Read the model definition and answer for the solid it produces. Units are mm, in the model's axes. Face numbers are marked on the shaded views. Coordinates: 2 decimals unless noted, no trailing zeros. Loops run counter-clockwise (first coordinate to the right, second up) from the corner with the lowest first, then second, coordinate; pieces in that order, holes last. Notation, with made-up numbers: (20.25, -11) - (30.25, -11) arc R21 ccw to (30.25, 18) - close; hole circle Ø1 at (78, 40.5). An arc over 180 degrees is marked (long way). Use one line per item in the form item = value. Start each with the question number.
1) Each of these flat-tipped pins is pushed along its axis until it touches: P1, Ø10, axis at x = -0.5, y = 4.5, coming from the -Z side; P2, Ø1.5, axis at y = -2.5, z = 3.5, coming from the -X side. Where does it stop, or does it pass through?
2) Consider line 1 (Y direction, x = 0, z = 2.7); line 2 (X direction, y = 2, z = 1.3); line 3 (X direction, y = 4.75, z = 2.05). Determine where each line is inside the solid, lowest interval first.
3) The mould has two halves that part along X. Classify the marked faces 1 and 2: released by +X, released by -X, zero draft, split by the parting line, or undercut.
4) A cutting plane is placed at A-A (y = 0). Give the vertices of the cut face in (x, z).
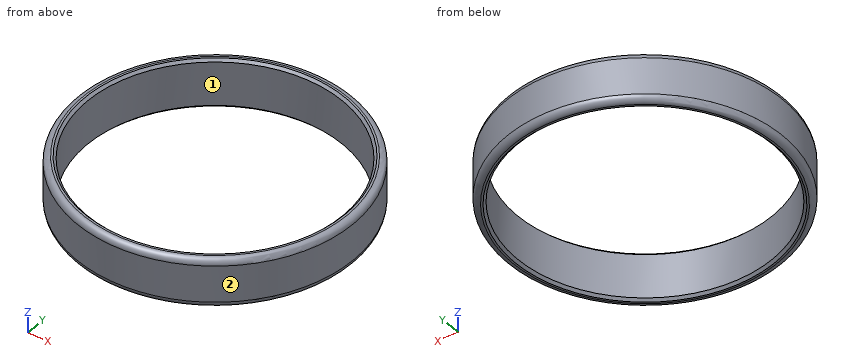
from build123d import *

# Parameters (mm, degrees)
F0_R     = 11.365202
F0_R_2   = 10.5
F1_DEPTH = 4
F2_R     = 0.5
F3_SIZE  = 0.2


with BuildPart() as f1:
    # F0 (on Top) → F1 (new body)
    with BuildSketch(Plane.XY):
        Circle(F0_R)
        Circle(F0_R_2, mode=Mode.SUBTRACT)
    extrude(amount=F1_DEPTH)

    # F2
    f2_edges = [f1.edges().sort_by_distance(p)[0] for p in [
        (-11.365202, 0, 0),
        (-11.365202, 0, 4),
    ]]
    fillet(f2_edges, radius=F2_R)

    # F3
    f3_edges = [f1.edges().sort_by_distance(p)[0] for p in [
        (-10.5, 0, 0),
        (-10.5, 0, 4),
    ]]
    chamfer(f3_edges, length=F3_SIZE)


solid = f1.part
Found:
q1.P1 = through
q1.P2 = -11.23
q2.line_1 = -11.37 to -10.5, 10.5 to 11.37
q2.line_2 = -11.19 to -10.31, 10.31 to 11.19
q2.line_3 = -10.32 to -9.36, 9.36 to 10.32
q3.face_1 = undercut
q3.face_2 = split by the parting line
q4.outline = (-11.37, 0.5) arc R0.5 ccw to (-10.87, 0) - (-10.7, 0) - (-10.5, 0.2) - (-10.5, 3.8) - (-10.7, 4) - (-10.87, 4) arc R0.5 ccw to (-11.37, 3.5) - close; (10.5, 0.2) - (10.7, 0) - (10.87, 0) arc R0.5 ccw to (11.37, 0.5) - (11.37, 3.5) arc R0.5 ccw to (10.87, 4) - (10.7, 4) - (10.5, 3.8) - close
